Check sheet for the modelled part. Datum: model origin and axes. Units: mm. Face numbers are marked on the shaded views. A direction names the side the tool comes from. Give positions to 0.01 mm unless a question says otherwise; leave off trailing zeros. Order: outer loops, then holes, each group sorted by start corner. A loop starts at its lowest first (then second) coordinate and runs counter-clockwise, first axis right, second up.
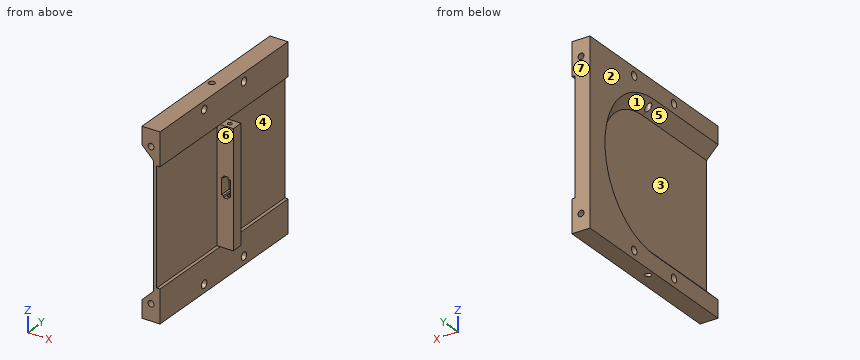
from build123d import *

# Parameters (mm, degrees)
SKETCH2_W              = 11
SKETCH2_H              = 116
BOSS_EXTRUDE2_DEPTH    = 109.999999964
SKETCH3_W              = 2
SKETCH3_H              = 70
CUT_EXTRUDE1_DEPTH     = 129.848748531
CUT_EXTRUDE2_DEPTH     = 7
CUT_EXTRUDE2_DRAFT     = -45
SKETCH6_W              = 70
SKETCH6_H              = 7
BOSS_EXTRUDE3_DEPTH    = 10
SKETCH7_R              = 1.27
CUT_EXTRUDE3_DEPTH     = 108.633637835
CUT_EXTRUDE4_DEPTH     = 84.23610994
CUT_EXTRUDE5_START     = -109.999999964
CUT_EXTRUDE5_OUTLINE_R = 1.8415
CUT_EXTRUDE5_DEPTH     = 109.999999964
SKETCH10_R             = 1.8415
CUT_EXTRUDE6_DEPTH     = 25.4
CUT_EXTRUDE7_START     = -25.4
SKETCH11_R             = 1.8415
CUT_EXTRUDE7_DEPTH     = 25.4
SKETCH12_R             = 2.413
CUT_EXTRUDE8_DEPTH     = 81.684571085


# Read off the part's stored shape, not the designer's step: Cut-Extrude5
with BuildPart() as part:
    # Sketch2 → Boss-Extrude2 (new body)
    with BuildSketch(Plane.XY.offset(54.999999982)):
        with Locations((-5.5, 0)):
            Rectangle(SKETCH2_W, SKETCH2_H)
    extrude(amount=-BOSS_EXTRUDE2_DEPTH)

    # Sketch3 → Cut-Extrude1 (cut, through all)
    with BuildSketch(Plane(origin=(0, 58, 0), x_dir=(1, 0, 0), z_dir=(0, 1, 0))):
        with Locations((-1, 1.8e-08)):
            Rectangle(SKETCH3_W, SKETCH3_H)
    extrude(amount=-CUT_EXTRUDE1_DEPTH, mode=Mode.SUBTRACT)


with BuildPart() as cut_extrude2_tool:
    # Sketch5 → Cut-Extrude2 (with draft: the straight prism first)
    with BuildSketch(Plane.ZY.offset(11)):
        with BuildLine():
            Line((-44.45, 0), (-44.45, -77.05))
            Line((-44.45, -77.05), (44.45, -77.05))
            Line((44.45, -77.05), (44.45, 0))
            ThreePointArc((44.45, 0), (0, 44.45), (-44.45, 0))
        make_face()
    extrude(amount=-CUT_EXTRUDE2_DEPTH)
    # Cut-Extrude2: the draft: its side faces are tilted about the plane it starts from
    cut_extrude2_sides = [cut_extrude2_tool.faces().sort_by_distance(p)[0] for p in [
        (-7.5, -38.525, -44.45),
        (-7.5, -77.05, 0),
        (-7.5, -38.525, 44.45),
        (-7.5, 44.45, 0),
    ]]
    draft(cut_extrude2_sides, Plane.ZY.offset(11), CUT_EXTRUDE2_DRAFT)


with BuildPart() as part_1:
    add(part.part)

    # Cut-Extrude2: cut by cut_extrude2_tool
    add(cut_extrude2_tool.part, mode=Mode.SUBTRACT)

    # Sketch6 → Boss-Extrude3 (add)
    with BuildSketch(Plane(origin=(-2, 0, 0), x_dir=(0, 0, -1), z_dir=(1, 0, 0))):
        with Locations((1.8e-08, 0)):
            Rectangle(SKETCH6_W, SKETCH6_H)
    extrude(amount=BOSS_EXTRUDE3_DEPTH)

    # Sketch7 → Cut-Extrude3 (cut, through all)
    with BuildSketch(Plane.XY.offset(34.999999982)):
        with Locations((3.5, 0)):
            Circle(SKETCH7_R)
    extrude(amount=-CUT_EXTRUDE3_DEPTH, mode=Mode.SUBTRACT)

    # Sketch8 → Cut-Extrude4 (cut, through all)
    with BuildSketch(Plane(origin=(0, 3.5, 0), x_dir=(1, 0, 0), z_dir=(0, 1, 0))):
        Polygon((0.75, 5), (0.75, -5), (2.103, -5), (2.103, -6.27), (4.897, -6.27), (4.897, -5), (6.25, -5), (6.25, 5), (4.897, 5), (4.897, 6.27), (2.103, 6.27), (2.103, 5), align=None)
    extrude(amount=-CUT_EXTRUDE4_DEPTH, mode=Mode.SUBTRACT)

    # Cut-Extrude5 outline → Cut-Extrude5 (cut)
    with BuildSketch(Plane.XY.offset(54.999999982).offset(CUT_EXTRUDE5_START)):
        with Locations((-7.5, 0)):
            Circle(CUT_EXTRUDE5_OUTLINE_R)
    extrude(amount=CUT_EXTRUDE5_DEPTH, mode=Mode.SUBTRACT)

    # Sketch10 → Cut-Extrude6 (cut)
    with BuildSketch(Plane(origin=(0, 58, 0), x_dir=(1, 0, 0), z_dir=(0, 1, 0))):
        with Locations(Location((-5.5, -44.999999982, 0), (0, 0, 270))):
            Circle(SKETCH10_R)
        with Locations(Location((-5.5, 44.999999982, 0), (0, 0, 270))):
            Circle(SKETCH10_R)
    extrude(amount=-CUT_EXTRUDE6_DEPTH, mode=Mode.SUBTRACT)

    # Sketch11 → Cut-Extrude7 (cut)
    with BuildSketch(Plane.XZ.offset(58).offset(CUT_EXTRUDE7_START)):
        with Locations(Location((-5.5, 44.999999982, 0), (0, 0, 90))):
            Circle(SKETCH11_R)
        with Locations(Location((-5.5, -44.999999982, 0), (0, 0, 90))):
            Circle(SKETCH11_R)
    extrude(amount=CUT_EXTRUDE7_DEPTH, mode=Mode.SUBTRACT)

    # Sketch12 → Cut-Extrude8 (cut, through all)
    with BuildSketch(Plane(origin=(0, 0, 0), x_dir=(0, 0, -1), z_dir=(1, 0, 0))):
        with Locations(Location((-49.999999982, 18, 0), (0, 0, 90))):
            Circle(SKETCH12_R)
        with Locations(Location((-49.999999982, -18, 0), (0, 0, 90))):
            Circle(SKETCH12_R)
        with Locations(Location((49.999999982, -18, 0), (0, 0, 90))):
            Circle(SKETCH12_R)
        with Locations(Location((49.999999982, 18, 0), (0, 0, 90))):
            Circle(SKETCH12_R)
    extrude(amount=-CUT_EXTRUDE8_DEPTH, mode=Mode.SUBTRACT)


solid = part_1.part
1) Section check A-A, the plane z = -50. Record the cut outline in (x, y), then the cut area to 3 significant figures.
Recorded:
outline: (-11, -58) - (0, -58) - (0, -20.41) - (-11, -20.41) - close; (-11, -15.59) - (0, -15.59) - (0, 15.59) - (-11, 15.59) - close; (-11, 20.41) - (0, 20.41) - (0, 58) - (-11, 58) - close; hole circle Ø3.68 at (-7.5, 0)
area: 1,160 mm2
2) Section check C-C, the plane y = -9.5. Record the cut outline in (x, z), then the cut area to 3 significant figures.
Recorded:
outline: (-11, -55) - (0, -55) - (0, -35) - (-2, -35) - (-2, 35) - (0, 35) - (0, 55) - (-11, 55) - (-11, 44.45) - (-4, 37.45) - (-4, -37.45) - (-11, -44.45) - close
area: 497 mm2
3) Draft check along Z on the marked faces 1, 2 and 3. Enter one of: +Z half, -Z half, draft (parallel to the pull), parting line (faces both ways), or undercut.
Recorded:
face 1: undercut
face 2: draft
face 3: undercut
4) Depth check by flat-ended pin: pin 1 Ø3 at (x, z) = (-5.5, 45) entering from +Y; pin 2 Ø5.5 at (x, y) = (2.5, -1) entering from +Z; pin 3 Ø8 at (y, z) = (-12, -2.5) entering from -X; pin 4 Ø12 at (y, z) = (-45, -36.5) entering from -X. Enter the tip coordinate at first touch or a pass-through.
Recorded:
pin 1: stops at y = 32.6
pin 2: stops at z = 55
pin 3: stops at x = -4
pin 4: stops at x = -9.05
5) Set-up check for the marked faces 4, 5, 6 and 7: record each of +Z, -Z, +X, -X, +Y, -Y from which the full face is reachable in a straight line by a thin tool's end or side.
Recorded:
face 4: +X, +Y
face 5: -X, -Y
face 6: +X, -Y
face 7: +Z, -Z, +X, -X, +Y
6) Section check D-D, the plane y = -40. Record the cut outline in (x, z), then the cut area to 3 significant figures.
Recorded:
outline: (-11, -55) - (0, -55) - (0, -35) - (-2, -35) - (-2, 35) - (0, 35) - (0, 55) - (-11, 55) - (-11, 44.45) - (-4, 37.45) - (-4, -37.45) - (-11, -44.45) - close; hole circle Ø3.68 at (-5.5, -45); hole circle Ø3.68 at (-5.5, 45)
area: 475 mm2
7) Material ranges on L1, parallel to Y at x = -3.5, z = 50; L2, parallel to X at y = -47, z = 45; L3, parallel to Z at x = -6.75, y = 18, recorded low to high.
Recorded:
L1: y = -58 to -20.41, -15.59 to 15.59, 20.41 to 58
L2: x = -11 to -7.34, -3.66 to 0
L3: z = -55 to -52.41, -47.59 to -35.94, 35.94 to 47.59, 52.41 to 55
8) Section check B-B, the plane y = 48. Record the cut outline in (x, z), then the cut area to 3 significant figures.
Recorded:
outline: (-11, -55) - (0, -55) - (0, -35) - (-2, -35) - (-2, 35) - (0, 35) - (0, 55) - (-11, 55) - close; hole circle Ø3.68 at (-5.5, -45); hole circle Ø3.68 at (-5.5, 45)
area: 1,050 mm2
